Design review of the part shown in the three views and the two pictorial views. Dimensions are in mm from the part's minimum x, y and z. A direction names the side the tool comes from. Give positions to 0.01 mm unless a question says otherwise; leave off trailing zeros. Write each loop counter-clockwise with the first axis right and the second up, starting at its lowest first coordinate (ties: lowest second). Pieces come first, ordered by that corner, then holes. Notation, with made-up numbers: M -17.5,-32.75 L 26.5,-32.75 A23 ccw 26.5,-7.75 Z; hole C 21.5,-26.5 d4. An arc over 180 degrees is marked long. Use one line per item in the form item = value. Start each with the question number.
Q1. For probe 1 along Y at (x, z) = (21, 9.5); probe 2 along Y at (x, z) = (29.5, 39); probe 3 along Y at (x, z) = (25, 11), list the stretches that pass through material, from the lowest coordinate up. Write a range as [from, to].
Q2. Mouldability with a two-part tool opening along X and no side actions: class the marked faces 4, 5, 6 and 7 as released by +X, released by -X, zero draft, split by the parting line, or undercut.
Q3. Consider section C-C on z = 29. Write out the cut boundary in (x, y).
Q4. Consider section D-D on y = 7. Write out the cut boundary in (x, z), and give its area (3 significant figures).
Q5. Consider section B-B on y = 18.5. Write out the cut boundary in (x, z).
Q6. Clearance check with flat-ended pins moving along their axes: pin 1 Ø10.5 at (x, z) = (22.5, 19.5) entering from +Y; pin 2 Ø1.7 at (x, y) = (23.5, 36) entering from +Z. State where each tip first meets the part, or that it passes through.
Q7. Tool access review of the marked faces 1, 2 and 3: name each direction out of +Z, -Z, +X, -X, +Y, -Y from which nothing blocks a thin tool from reaching the whole face with its end or side.
Q8. Consider section A-A on x = 21. Write out the cut boundary in (y, z).
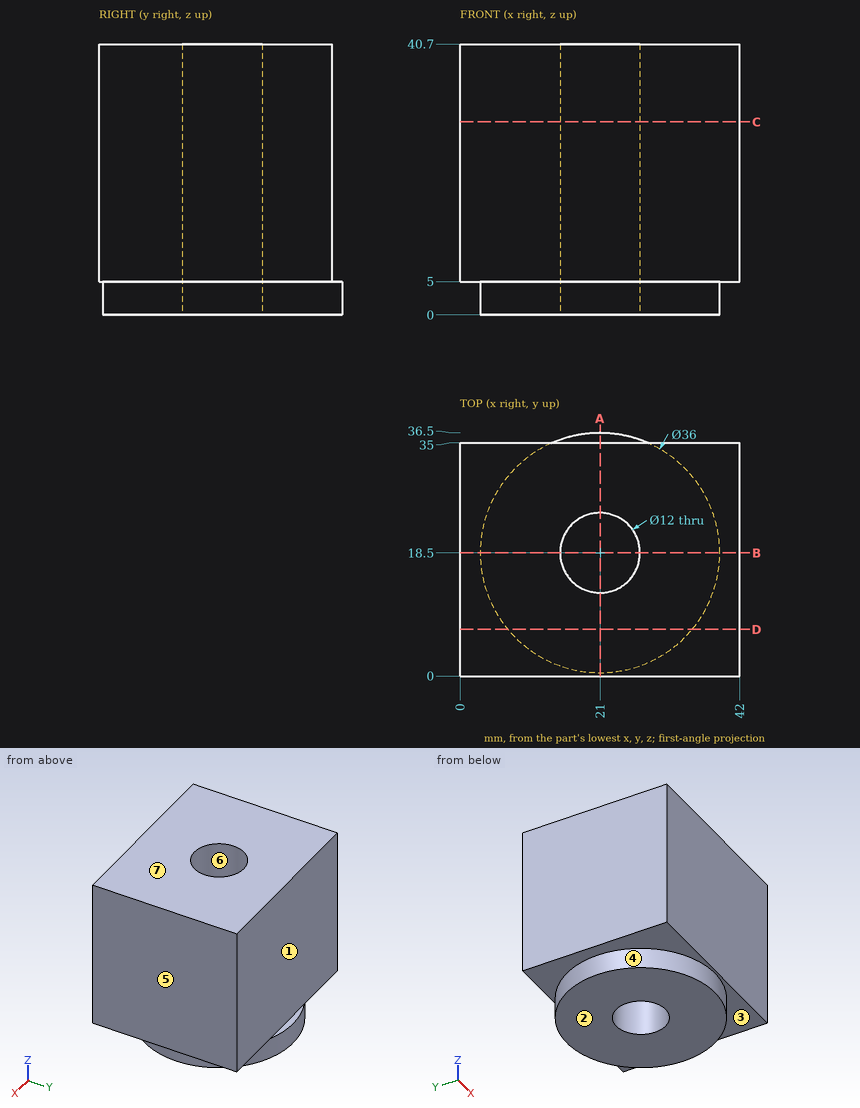
Working result:
q1.probe_1 = [0, 12.5], [24.5, 35]
q1.probe_2 = [0, 35]
q1.probe_3 = [0, 14.03], [22.97, 35]
q2.face_4 = split by the parting line
q2.face_5 = released by +X
q2.face_6 = undercut
q2.face_7 = zero draft
q3.outline = M 0,0 L 42,0 L 42,35 L 0,35 Z; hole C 21,18.5 d12
q4.outline = M 0,5 L 7.15,5 L 7.15,0 L 34.85,0 L 34.85,5 L 42,5 L 42,40.7 L 0,40.7 Z
q4.area = 1,640 mm²
q5.outline = M 0,5 L 3,5 L 3,0 L 15,0 L 15,40.7 L 0,40.7 Z; M 27,0 L 39,0 L 39,5 L 42,5 L 42,40.7 L 27,40.7 Z
q6.pin_1 = 35
q6.pin_2 = 5
q7.face_1 = +Z, +X, -X, +Y
q7.face_2 = -Z, +X, -X, +Y, -Y
q7.face_3 = -Z
q8.outline = M 0,5 L 0.5,5 L 0.5,0 L 12.5,0 L 12.5,40.7 L 0,40.7 Z; M 24.5,0 L 36.5,0 L 36.5,5 L 35,5 L 35,40.7 L 24.5,40.7 Z
